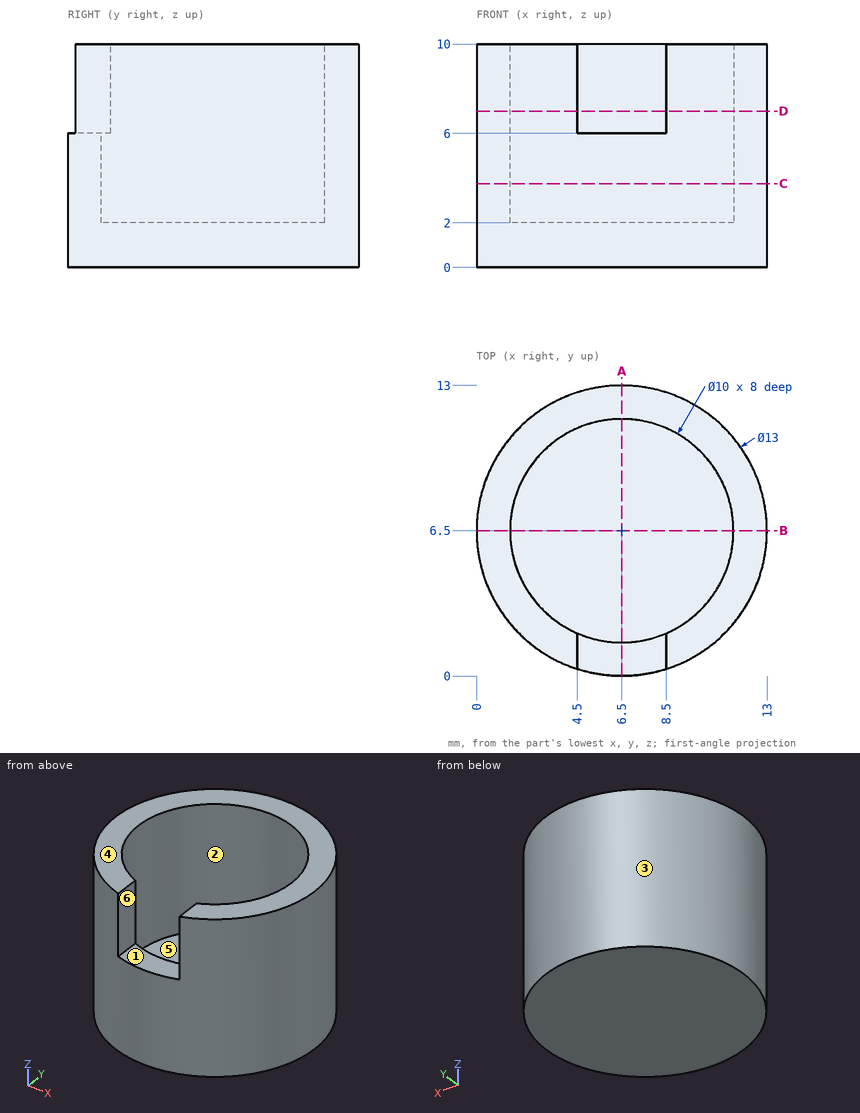
Design review of the part shown in the three views and the two pictorial views. Dimensions are in mm from the part's minimum x, y and z. A direction names the side the tool comes from. Round coordinates to 2 decimals unless told otherwise and drop trailing zeros. Order: outer loops, then holes, each group sorted by start corner. A loop starts at its lowest first (then second) coordinate and runs counter-clockwise, first axis right, second up.
Item 1: Add section B-B, the plane y = 6.5. State the section outline as (x, z) points.
Working result:
outline: (0, 0) - (13, 0) - (13, 10) - (11.5, 10) - (11.5, 2) - (1.5, 2) - (1.5, 10) - (0, 10) - close
Item 2: Machinability: for the marked faces 4, 5 and 6, which of the approach directions +Z, -Z, +X, -X, +Y, -Y give a long, thin tool a straight path to every point of the face, cutting with its end or side? Answer none if there is none.
Working result:
face 4: +Z, +X, -X, +Y, -Y
face 5: +Z
face 6: +Z, -Y
Item 3: Add section A-A, the plane x = 6.5. State the section outline as (y, z) points, and give its area (3 significant figures).
Working result:
outline: (0, 0) - (13, 0) - (13, 10) - (11.5, 10) - (11.5, 2) - (1.5, 2) - (1.5, 6) - (0, 6) - close
area: 44.0 mm2
Item 4: Add section C-C, the plane z = 3.75. State the section outline as (x, y) points, and give its area (3 significant figures).
Working result:
outline: circle Ø13 at (6.5, 6.5); hole circle Ø10 at (6.5, 6.5)
area: 54.2 mm2
Item 5: For pin 1 (3 mm diameter, centred on x = 2, z = 3.5, fed in from +Y); pin 2 (5 mm diameter, centred on x = 6.5, y = 2.5, fed in from +Z); pin 3 (0.5 mm diameter, centred on y = 1, z = 8.5, fed in from +X); pin 4 (3 mm diameter, centred on y = 3.5, z = 5.5, fed in from +X), all flat-tipped, find the tip position at first contact; note any pin that passes through.
Working result:
pin 1: stops at y = 12.27
pin 2: stops at z = 10
pin 3: stops at x = 10.33
pin 4: stops at x = 12.82
Item 6: To check wall thickness, follow probe 1 along X at (y, z) = (6.5, 5); probe 2 along Z at (x, y) = (2.25, 7.25). State the ranges of each line that lie inside material, in increasing order.
Working result:
probe 1: x = 0 to 1.5, 11.5 to 13
probe 2: z = 0 to 2
Item 7: Add section D-D, the plane z = 7. State the section outline as (x, y) points.
Working result:
outline: (4.5, 0.32) - (4.5, 1.92) arc R5 cw (long way) to (8.5, 1.92) - (8.5, 0.32) arc R6.5 ccw (long way) to start
Item 8: Draft analysis for pull direction Y (two halves, no side actions). For the marked faces 1, 2 and 3, state which applies: released by +Y, released by -Y, zero draft, split by the parting line, or undercut.
Working result:
face 1: zero draft
face 2: undercut
face 3: split by the parting line
